from build123d import *

# Parameters (mm, degrees)
SALIENTE_EXTRUIR1_DEPTH = 40
CORTAR_EXTRUIR1_REACH   = 71.282
CROQUIS2_R              = 2.25
SALIENTE_EXTRUIR2_DEPTH = 20
CROQUIS5_R              = 4.15
CORTAR_EXTRUIR2_DEPTH   = 25
REDONDEO2_R             = 4
CORTAR_EXTRUIR3_REACH   = 72.887
CROQUIS10_R             = 4.5
CROQUIS10_R_2           = 2.25
CORTAR_EXTRUIR5_START   = -20
CORTAR_EXTRUIR5_DEPTH   = 20
CORTAR_EXTRUIR6_DEPTH   = 5.5
CORTAR_EXTRUIR7_DEPTH   = 1


with BuildPart() as part:
    # Croquis1 → Saliente-Extruir1 (new body)
    with BuildSketch(Plane(origin=(0, 0, 0), x_dir=(1, 0, 0), z_dir=(0, 1, 0))):
        Polygon((0, 0), (40, 0), (40, 20), (20, 20), (20, 40), (0, 40), align=None)
    extrude(amount=SALIENTE_EXTRUIR1_DEPTH)

    # Croquis2 → Cortar-Extruir1 (cut, up to next)
    with BuildSketch(Plane(origin=(0, 40, 0), x_dir=(1, 0, 0), z_dir=(0, 1, 0)), mode=Mode.PRIVATE) as cortar_extruir1_sk1:
        with Locations(Location((30, 10, 0), (0, 0, 270))):
            Circle(CROQUIS2_R)
    cortar_extruir1_tool1 = extrude(cortar_extruir1_sk1.sketch, amount=-CORTAR_EXTRUIR1_REACH, mode=Mode.PRIVATE) & part.part
    # Croquis2 → Cortar-Extruir1 (cut, up to next)
    with BuildSketch(Plane(origin=(0, 40, 0), x_dir=(1, 0, 0), z_dir=(0, 1, 0)), mode=Mode.PRIVATE) as cortar_extruir1_sk2:
        with Locations(Location((10, 10, 0), (0, 0, 270))):
            Circle(CROQUIS2_R)
    cortar_extruir1_tool2 = extrude(cortar_extruir1_sk2.sketch, amount=-CORTAR_EXTRUIR1_REACH, mode=Mode.PRIVATE) & part.part
    add(cortar_extruir1_tool1.solids().sort_by_distance((30, 40, -10))[0], mode=Mode.SUBTRACT)
    add(cortar_extruir1_tool2.solids().sort_by_distance((10, 40, -10))[0], mode=Mode.SUBTRACT)

    # Croquis3 → Saliente-Extruir2 (add)
    with BuildSketch(Plane.ZY):
        with BuildLine():
            Line((35, 40), (0, 40))
            Line((0, 40), (0, 0))
            Line((0, 0), (35, 0))
            ThreePointArc((35, 0), (55, 20), (35, 40))
        make_face()
    extrude(amount=-SALIENTE_EXTRUIR2_DEPTH)

    # Croquis5 → Cortar-Extruir2 (cut)
    with BuildSketch(Plane(origin=(0, 0, -40), x_dir=(-1, 0, 0), z_dir=(0, 0, -1))):
        with Locations((-10, 30)):
            Circle(CROQUIS5_R)
    extrude(amount=-CORTAR_EXTRUIR2_DEPTH, mode=Mode.SUBTRACT)

    # Redondeo2
    redondeo2_edges = [part.edges().sort_by_distance(p)[0] for p in [
        (0, 20, -40),
        (20, 20, -40),
        (20, 20, -20),
        (40, 20, -20),
        (40, 20, 0),
        (20, 20, 0),
    ]]
    fillet(redondeo2_edges, radius=REDONDEO2_R)

    # Croquis10 → Cortar-Extruir3 (cut, up to next)
    with BuildSketch(Plane(origin=(20, 0, 0), x_dir=(0, 0, -1), z_dir=(1, 0, 0)), mode=Mode.PRIVATE) as cortar_extruir3_sk1:
        with Locations((-29.5, 20)):
            Circle(CROQUIS10_R)
    cortar_extruir3_tool1 = extrude(cortar_extruir3_sk1.sketch, amount=-CORTAR_EXTRUIR3_REACH, mode=Mode.PRIVATE) & part.part
    # Croquis10 → Cortar-Extruir3 (cut, up to next)
    with BuildSketch(Plane(origin=(20, 0, 0), x_dir=(0, 0, -1), z_dir=(1, 0, 0)), mode=Mode.PRIVATE) as cortar_extruir3_sk2:
        with Locations((-14, 20)):
            Circle(CROQUIS10_R_2)
    cortar_extruir3_tool2 = extrude(cortar_extruir3_sk2.sketch, amount=-CORTAR_EXTRUIR3_REACH, mode=Mode.PRIVATE) & part.part
    # Croquis10 → Cortar-Extruir3 (cut, up to next)
    with BuildSketch(Plane(origin=(20, 0, 0), x_dir=(0, 0, -1), z_dir=(1, 0, 0)), mode=Mode.PRIVATE) as cortar_extruir3_sk3:
        with Locations((-45, 20)):
            Circle(CROQUIS10_R_2)
    cortar_extruir3_tool3 = extrude(cortar_extruir3_sk3.sketch, amount=-CORTAR_EXTRUIR3_REACH, mode=Mode.PRIVATE) & part.part
    add(cortar_extruir3_tool1.solids().sort_by_distance((20, 20, 29.5))[0], mode=Mode.SUBTRACT)
    add(cortar_extruir3_tool2.solids().sort_by_distance((20, 20, 14))[0], mode=Mode.SUBTRACT)
    add(cortar_extruir3_tool3.solids().sort_by_distance((20, 20, 45))[0], mode=Mode.SUBTRACT)

    # Croquis12 → Cortar-Extruir5 (cut)
    with BuildSketch(Plane(origin=(20, 0, 0), x_dir=(0, 0, -1), z_dir=(1, 0, 0)).offset(CORTAR_EXTRUIR5_START)):
        with BuildLine():
            Line((-15.1, 22.25), (-12.9, 22.25))
            ThreePointArc((-12.9, 22.25), (-10.65, 20), (-12.9, 17.75))
            Line((-12.9, 17.75), (-15.1, 17.75))
            ThreePointArc((-15.1, 17.75), (-17.35, 20), (-15.1, 22.25))
        make_face()
        with BuildLine():
            Line((-43.9, 17.75), (-46.1, 17.75))
            ThreePointArc((-46.1, 17.75), (-48.35, 20), (-46.1, 22.25))
            Line((-46.1, 22.25), (-43.9, 22.25))
            ThreePointArc((-43.9, 22.25), (-41.65, 20), (-43.9, 17.75))
        make_face()
    extrude(amount=CORTAR_EXTRUIR5_DEPTH, mode=Mode.SUBTRACT)

    # Croquis14 → Cortar-Extruir6 (cut)
    with BuildSketch(Plane(origin=(20, 0, 0), x_dir=(0, 0, -1), z_dir=(1, 0, 0))):
        with BuildLine():
            Line((-48.021686747, 25.472396189), (-33.243975904, 30.661737402))
            ThreePointArc((-33.243975904, 30.661737402), (-29.5, 31.3), (-25.756024096, 30.661737402))
            Line((-25.756024096, 30.661737402), (-10.978313253, 25.472396189))
            ThreePointArc((-10.978313253, 25.472396189), (-7.1, 20), (-10.978313253, 14.527603811))
            Line((-10.978313253, 14.527603811), (-25.756024096, 9.338262598))
            ThreePointArc((-25.756024096, 9.338262598), (-29.5, 8.7), (-33.243975904, 9.338262598))
            Line((-33.243975904, 9.338262598), (-48.021686747, 14.527603811))
            ThreePointArc((-48.021686747, 14.527603811), (-51.9, 20), (-48.021686747, 25.472396189))
        make_face()
    extrude(amount=-CORTAR_EXTRUIR6_DEPTH, mode=Mode.SUBTRACT)

    # Croquis15 → Cortar-Extruir7 (cut)
    with BuildSketch(Plane(origin=(0, 40, 0), x_dir=(1, 0, 0), z_dir=(0, 1, 0))):
        with BuildLine():
            Line((11.307692308, -8.153846154), (11.846153846, -8.153846154))
            add(Edge.make_bspline(
                [(11.846153846, -8.153846154), (11.842645038, -8.225282314), (11.835753833, -8.36558103), (11.803468313, -8.570131316), (11.757314544, -8.765671861), (11.691903885, -8.950526266), (11.611127437, -9.126902771), (11.512233689, -9.292459299), (11.397330895, -9.448838982), (11.266629849, -9.593081031), (11.124807169, -9.724936298), (10.972712592, -9.840005009), (10.811909364, -9.936114468), (10.643792222, -10.016896686), (10.466416843, -10.077459923), (10.281478736, -10.12241659), (10.088142, -10.149460313), (9.956416396, -10.152367573), (9.889423077, -10.153846154)],
                knots=[0, 0, 0, 0, 1.100776268, 2.161895295, 3.184016182, 4.190939212, 5.176500551, 6.166955529, 7.155448256, 8.160289653, 9.16017456, 10.133824356, 11.091467644, 12.04088621, 13.000931625, 13.972173743, 14.968683325, 16, 16, 16, 16], degree=3))
            add(Edge.make_bspline(
                [(9.889423077, -10.153846154), (9.823627463, -10.152318442), (9.694341431, -10.149316542), (9.50572919, -10.123149389), (9.325747878, -10.08305056), (9.15643722, -10.023630413), (8.996059613, -9.949071125), (8.846600799, -9.856346883), (8.704446708, -9.749845084), (8.576574014, -9.62422099), (8.459107518, -9.490179765), (8.357858501, -9.347024863), (8.270662051, -9.198998287), (8.19929448, -9.044943733), (8.145194688, -8.884359526), (8.105111926, -8.71878524), (8.082198454, -8.546310036), (8.078701137, -8.429552583), (8.076923077, -8.370192308)],
                knots=[0, 0, 0, 0, 1.111674182, 2.184400057, 3.212814286, 4.223731311, 5.211378316, 6.196328225, 7.191884489, 8.207283132, 9.220262353, 10.201199469, 11.166417575, 12.120932471, 13.06540007, 14.026332106, 14.996573967, 16, 16, 16, 16], degree=3))
            add(Edge.make_bspline(
                [(8.076923077, -8.370192308), (8.079825859, -8.286624627), (8.085580483, -8.120955761), (8.13480446, -7.877501183), (8.211686738, -7.641628758), (8.304245432, -7.451786912), (8.397645126, -7.298829691), (8.481727628, -7.172830092), (8.580719899, -7.037198101), (8.693776191, -6.891384748), (8.822843495, -6.737299583), (8.964568659, -6.571798854), (9.122611785, -6.397942783), (9.233438011, -6.279119385), (9.290865385, -6.217548077)],
                knots=[0, 0, 0, 0, 1.184416499, 2.348048165, 3.509039915, 4.696071444, 5.333504901, 6.05069495, 6.844171097, 7.714965912, 8.667477798, 9.695072654, 10.805644396, 12, 12, 12, 12], degree=3))
            Line((9.290865385, -6.217548077), (10.792067308, -4.615384615))
            Line((10.792067308, -4.615384615), (8, -4.615384615))
            Line((8, -4.615384615), (8, -4))
            Line((8, -4), (12.076923077, -4))
            Line((12.076923077, -4), (9.75, -6.483173077))
            add(Edge.make_bspline(
                [(9.75, -6.483173077), (9.693342469, -6.542309805), (9.584514946, -6.655899358), (9.430654729, -6.82178687), (9.292241226, -6.975502303), (9.169182624, -7.117726807), (9.061377669, -7.2476541), (8.969171289, -7.366302394), (8.892155948, -7.472653483), (8.810535736, -7.597590295), (8.732705448, -7.750311776), (8.664300588, -7.936006624), (8.622889216, -8.127587641), (8.617896164, -8.257013212), (8.615384615, -8.322115385)],
                knots=[0, 0, 0, 0, 1.329530082, 2.553755191, 3.672934919, 4.687409497, 5.60679272, 6.413407421, 7.126401618, 7.737995624, 8.834647426, 9.90044882, 10.943907757, 12, 12, 12, 12], degree=3))
            add(Edge.make_bspline(
                [(8.615384615, -8.322115385), (8.616463264, -8.363059449), (8.618589075, -8.443752337), (8.637705753, -8.561983012), (8.665791949, -8.676472493), (8.709081452, -8.7858052), (8.761092196, -8.892131494), (8.827539757, -8.992218726), (8.903471871, -9.089478629), (8.991549398, -9.180576241), (9.088242157, -9.264035799), (9.190407045, -9.337961219), (9.298492072, -9.399742965), (9.4120468, -9.45038885), (9.530753256, -9.490118105), (9.654841407, -9.51764709), (9.783968288, -9.53493135), (9.872139995, -9.53726993), (9.917067308, -9.538461538)],
                knots=[0, 0, 0, 0, 0.991504627, 1.954065223, 2.895985987, 3.842598665, 4.797835564, 5.759220273, 6.74786863, 7.784730864, 8.824135544, 9.839918996, 10.835834653, 11.835434876, 12.84861661, 13.863796685, 14.911511676, 16, 16, 16, 16], degree=3))
            add(Edge.make_bspline(
                [(9.917067308, -9.538461538), (9.964000721, -9.537284508), (10.056170195, -9.534973014), (10.191204591, -9.5174538), (10.320924626, -9.490921844), (10.443331351, -9.448683187), (10.560986519, -9.399248357), (10.67088869, -9.335238949), (10.776125151, -9.262098301), (10.874580094, -9.17682095), (10.964251271, -9.080555667), (11.045825943, -8.975772607), (11.114944972, -8.860614179), (11.176301237, -8.737843643), (11.223226665, -8.604087986), (11.263344544, -8.462618365), (11.29248559, -8.311416341), (11.302539212, -8.20724191), (11.307692308, -8.153846154)],
                knots=[0, 0, 0, 0, 1.031072318, 2.024855787, 2.988461151, 3.935103592, 4.865765533, 5.788564469, 6.724086513, 7.67908574, 8.64457978, 9.611397706, 10.591395687, 11.591555111, 12.622101007, 13.700900657, 14.821571223, 16, 16, 16, 16], degree=3))
        make_face()
    extrude(amount=-CORTAR_EXTRUIR7_DEPTH, mode=Mode.SUBTRACT)


solid = part.part
Here's how the part is built. I have some questions about the finished solid (model axes, mm). A direction names the side the tool comes from. Coordinates: 2 decimals unless noted, no trailing zeros. Write each loop counter-clockwise with the first axis right and the second up, starting at its lowest first coordinate (ties: lowest second). Pieces come first, ordered by that corner, then holes.
Item 1: If I drill on line 1 (X direction, y = 12, z = -10); line 2 (Y direction, x = 10, z = -20); line 3 (Z direction, x = 11, y = 18), over which ranges is the centre line in solid material (lowest first)?
Item 2: I want a section at B-B on y = 36. Write out the boundary of the cut face in (x, z).
Item 3: On a 3-axis mill with a long thin cutter (end or side, diameter ignored), from which of +Z, -Z, +X, -X, +Y, -Y can I reach the whole of each face in a straight line? I mean faces 4 (the flat face through (7, 17.75, 14)), 5 (the cylindrical face through (13.059, 32.805, -27.675)), 6 (the flat face through (9, 39, 7)), 7 (the cylindrical face through (17.3, 20.1, 7.1)). Say none if no direction works.
Item 4: I want a section at D-D on z = 27.5. Write out the boundary of the cut face in (x, y), and give its area (3 significant figures).
Item 5: I want a section at C-C on x = 31. Write out the boundary of the cut face in (y, z).
Item 6: I want a section at A-A on z = -10. Write out the boundary of the cut face in (x, y), and give its area (3 significant figures).
Item 7: Will these pins go through, and if not, where does the flat tip stop? pin 1 (4 mm diameter, centred on x = 10, z = -10, fed in from -Y); pin 2 (13 mm diameter, centred on y = 15.5, z = -27.5, fed in from +X); pin 3 (1.8 mm diameter, centred on x = 8, z = 45.5, fed in from -Y); pin 4 (13.5 mm diameter, centred on x = 10, y = 30, fed in from -Z).
Item 8: If we mould it in two halves opening along Z, with no side actions, what happens to faces 1 (the flat face through (20, 29, 18)), 2 (the cylindrical face through (38.859, 20.28, -18.797)), 3 (the flat face through (7, 17.75, 45))? For each: +Z half, -Z half, draft (parallel to the pull), parting line (faces both ways), or undercut.
Findings below:
1. line 1: x = 0 to 7.75, 12.25 to 27.75, 32.25 to 40
1. line 2: y = 0 to 25.85, 34.15 to 40
1. line 3: z = -40 to -12.02, -7.98 to 11.87, 16.13 to 25.47, 33.53 to 42.87, 47.13 to 54.9
2. outline: (0, -36) arc R4 ccw to (4, -40) - (16, -40) arc R4 ccw to (20, -36) - (20, -24) arc R4 cw to (24, -20) - (36, -20) arc R4 ccw to (40, -16) - (40, -4) arc R4 ccw to (36, 0) - (24, 0) arc R4 cw to (20, 4) - (20, 47) - (0, 47) - close; hole circle Ø4.5 at (10, -10); hole circle Ø4.5 at (30, -10)
3. face 4: +X, -X
3. face 5: -Z
3. face 6: +Y
3. face 7: +X
4. outline: (0, 0) - (20, 0) - (20, 8.88) - (14.5, 8.88) - (14.5, 15.97) - (0, 15.97) - close; (0, 24.03) - (14.5, 24.03) - (14.5, 31.12) - (20, 31.12) - (20, 40) - (0, 40) - close
4. area: 561 mm2
5. outline: (0, -20) - (40, -20) - (40, -12.02) - (0, -12.02) - close; (0, -7.98) - (40, -7.98) - (40, 0) - (0, 0) - close
6. outline: (0, 0) - (7.75, 0) - (7.75, 40) - (0, 40) - close; (12.25, 0) - (27.75, 0) - (27.75, 40) - (12.25, 40) - close; (32.25, 0) - (40, 0) - (40, 40) - (32.25, 40) - close
6. area: 1,240 mm2
7. pin 1: passes through
7. pin 2: stops at x = 21.35
7. pin 3: stops at y = 2.45
7. pin 4: stops at z = -40
8. face 1: draft
8. face 2: -Z half
8. face 3: undercut
